CAD build for the part. Positions are in the model's coordinates, mm. A direction names the side the tool comes from. Coordinates: 2 decimals unless noted, no trailing zeros. Order: outer loops, then holes, each group sorted by start corner. A loop starts at its lowest first (then second) coordinate and runs counter-clockwise, first axis right, second up.
Autodesk Inventor part; units mm, degrees
ref_plane "YZ Plane" through (0, 0, 0) normal (1, 0, 0) x (0, 1, 0)
ref_plane "XZ Plane" through (0, 0, 0) normal (0, 1, 0) x (-1, 0, 0)
ref_plane "XY Plane" through (0, 0, 0) normal (0, 0, 1) x (1, 0, 0)
sketch "Sketch1" plane through (0, 0, 0) normal (0, 1, 0) x (-1, 0, 0)
  circle A0 centre (0, 0) radius 60
  dimension "d0" = 120
extrude "Extrusion1" add sketch "Sketch1" along normal blind 8
sketch "Sketch2" plane through (0, 8, 0) normal (0, 1, 0) x (1, 0, 0)
  circle A0 centre (-54, 0) radius 4
  circle A1 centre (-54, 0) radius 2.5
  circle A2 centre (0, -54) radius 4
  circle A3 centre (0, -54) radius 2.5
  circle A4 centre (54, 0) radius 4
  circle A5 centre (54, 0) radius 2.5
  circle A6 centre (0, 54) radius 4
  circle A7 centre (0, 54) radius 2.5
  point P0 (0, 0)
  dimension "d3" = 8
  dimension "d4" = 5
  dimension "d5" = 8
  dimension "d6" = 5
  dimension "d7" = 8
  dimension "d8" = 5
  dimension "d9" = 8
  dimension "d10" = 5
extrude "Extrusion2" cut sketch "Sketch2" against normal blind 8 contours A1 | A3 | A5 | A7
sketch "Sketch3" plane through (0, 8, 0) normal (0, 1, 0) x (1, 0, 0)
  circle A0 centre (-54, 0) radius 2.5
  circle A1 centre (-54, 0) radius 4
  circle A2 centre (-54, 0) radius 2.5
  circle A3 centre (0, 54) radius 2.5
  circle A4 centre (0, 54) radius 4
  circle A5 centre (0, 54) radius 2.5
  circle A6 centre (54, 0) radius 2.5
  circle A7 centre (54, 0) radius 4
  circle A8 centre (54, 0) radius 2.5
  circle A9 centre (0, -54) radius 4
  circle A10 centre (0, -54) radius 2.5
  point P0 (0, 0)
  dimension "d13" = 8
  dimension "d14" = 8
  dimension "d15" = 5
  dimension "d16" = 8
  dimension "d17" = 5
  dimension "d18" = 8
extrude "Extrusion3" cut sketch "Sketch3" against normal blind 3
sketch "Sketch4" plane through (0, 8, 0) normal (0, 1, 0) x (1, 0, 0)
  circle A0 centre (0, 0) radius 47.5
  circle A1 centre (0, 0) radius 45
  line L0 (0, 0) -> (-10, 0)
  line L1 (-10, 0) -> (-10, -9)
  line L2 (-10, -9) -> (0, -9)
  line L3 (0, -9) -> (0, 0)
  line L4 (0, -9) -> (10, -9)
  line L5 (10, -9) -> (10, 0)
  line L6 (10, 0) -> (0, 0)
  line L7 (0, 0) -> (0, -9)
  line L8 (-10, -9) -> (10, -9)
  line L9 (10, -9) -> (10, -16)
  line L10 (10, -16) -> (-10, -16)
  line L11 (-10, -16) -> (-10, -9)
  dimension "d21" = 95
  dimension "d22" = 90
  dimension "d23" = 10
  dimension "d24" = 9
  dimension "d25" = 10
  dimension "d26" = 7
extrude "Extrusion4" add sketch "Sketch4" along normal blind 10 contours A0
sketch "Sketch5" plane through (0, 8, 0) normal (0, 1, 0) x (1, 0, 0)
  line L0 (0, 0) -> (-10, 0)
  line L1 (-10, 0) -> (-10, -9)
  line L2 (-10, -9) -> (0, -9)
  line L3 (0, -9) -> (0, 0)
  line L4 (-10, -9) -> (10, -9)
  line L5 (10, -9) -> (10, -16)
  line L6 (10, -16) -> (-10, -16)
  line L7 (-10, -16) -> (-10, -9)
  line L8 (-10, -9) -> (10, -9)
  line L9 (10, -9) -> (10, 31)
  line L10 (10, 31) -> (-10, 31)
  line L11 (-10, 31) -> (-10, -9)
  line L12 (-10, 31) -> (-2, 31)
  line L13 (-2, 31) -> (-2, 38.36)
  line L14 (-2, 38.36) -> (-10, 38.36)
  line L15 (-10, 38.36) -> (-10, 31)
  line L16 (-10, 31) -> (10, 31)
  line L17 (10, 31) -> (10, 39)
  line L18 (10, 39) -> (-10, 39)
  line L19 (-10, 39) -> (-10, 31)
  line L20 (-10, -9) -> (10, -9)
  line L21 (10, -9) -> (10, -17)
  line L22 (10, -17) -> (-10, -17)
  line L23 (-10, -17) -> (-10, -9)
  dimension "d29" = 10
  dimension "d30" = 9
  dimension "d31" = 20
  dimension "d32" = 7
  dimension "d33" = 40
  dimension "d34" = 8
  dimension "d35" = 8
  dimension "d36" = 8
extrude "Extrusion5" add sketch "Sketch5" along normal blind 28 contours L4 L5 L6 L7 L2 | L15 L14 L13 L10 | L6 L21 L22 L23 | L13 L14 L19 L18 L17 L10
sketch "Sketch6" plane through (0, 36, 0) normal (0, 1, 0) x (1, 0, 0)
  line L0 (10, -17) -> (-10, -17)
  line L1 (-10, -9) -> (10, -9)
  line L2 (0, -17) -> (-4, -17)
  line L3 (-4, -17) -> (-4, -9)
  line L4 (-4, -9) -> (0, -9)
  line L5 (0, -9) -> (0, -17)
  line L6 (0, -17) -> (4, -17)
  line L7 (4, -17) -> (4, -9)
  line L8 (4, -9) -> (0, -9)
  line L9 (0, -9) -> (0, -17)
  point P0 (0, 0)
  dimension "d39" = 4
  dimension "d40" = 4
extrude "Extrusion6" cut sketch "Sketch6" against normal blind 28
sketch "Sketch7" plane through (0, 36, 0) normal (0, 1, 0) x (1, 0, 0)
  line L0 (-10, -17) -> (-4, -17)
  line L1 (4, -9) -> (10, -9)
  line L2 (-4, -17) -> (4, -17)
  line L3 (4, -17) -> (4, -9)
  line L4 (4, -9) -> (-4, -9)
  line L5 (-4, -9) -> (-4, -17)
  point P0 (0, 0)
extrude "Extrusion7" add sketch "Sketch7" against normal blind 22
sketch "Sketch8" plane through (0, 36, 0) normal (0, 1, 0) x (1, 0, 0)
  line L0 (-4, -17) -> (-10, -17)
  line L1 (10, -17) -> (10, -9)
  line L2 (-10, -17) -> (10, -17)
  line L3 (10, -17) -> (10, -15)
  line L4 (10, -15) -> (-10, -15)
  line L5 (-10, -15) -> (-10, -17)
  line L6 (-4, -9) -> (4, -9)
  line L7 (0, -9) -> (-5, -9)
  line L8 (-5, -9) -> (-5, -17)
  line L9 (-5, -17) -> (0, -17)
  line L10 (0, -17) -> (0, -9)
  line L11 (-10, -17) -> (10, -17)
  line L12 (0, -9) -> (5, -9)
  line L13 (5, -9) -> (5, -17)
  line L14 (5, -17) -> (0, -17)
  line L15 (0, -17) -> (0, -9)
  circle A0 centre (-5, -15) radius 2
  circle A1 centre (5, -15) radius 2
  line L16 (-10, 31) -> (-10, 39)
  line L17 (10, 39) -> (10, 31)
  line L18 (-10, 39) -> (10, 39)
  line L19 (10, 39) -> (10, 37)
  line L20 (10, 37) -> (-10, 37)
  line L21 (-10, 37) -> (-10, 39)
  line L22 (10, 31) -> (-10, 31)
  line L23 (-10, 39) -> (10, 39)
  line L24 (0, 31) -> (-5, 31)
  line L25 (-5, 31) -> (-5, 39)
  line L26 (-5, 39) -> (0, 39)
  line L27 (0, 39) -> (0, 31)
  line L28 (0, 31) -> (5, 31)
  line L29 (5, 31) -> (5, 39)
  line L30 (5, 39) -> (0, 39)
  line L31 (0, 39) -> (0, 31)
  circle A2 centre (-5, 37) radius 2
  circle A3 centre (5, 37) radius 2
  point P0 (0, 0)
  dimension "d45" = 2
  dimension "d46" = 5
  dimension "d47" = 5
  dimension "d48" = 4
  dimension "d49" = 4
  dimension "d50" = 2
  dimension "d51" = 4
  dimension "d52" = 4
extrude "Extrusion8" cut sketch "Sketch8" against normal blind 10 contours A0 L4 L8 | L8 L4 A0 | L8 A0 L4 | L4 A0 L8 | A1 L4 L13 | L13 L4 A1 | L13 A1 L4 | L4 A1 L13 | A2 L25 L20 | L20 L25 A2 | L25 L20 A2 | A2 L20 L25 | A3 L20 L29 | L29 L20 A3 | A3 L29 L20 | A3 L20 L29
sketch "Sketch9" plane through (0, 36, 0) normal (0, 1, 0) x (1, 0, 0)
  line L0 (-10, -17) -> (-5, -17)
  line L1 (10, -9) -> (-10, -9)
  line L2 (-10, -17) -> (10, -17)
  line L3 (10, -17) -> (10, -9)
  line L4 (10, -9) -> (-10, -9)
  line L5 (-10, -9) -> (-10, -17)
  line L6 (10, 31) -> (10, 39)
  line L7 (-10, 31) -> (10, 31)
  line L8 (10, 31) -> (10, 39)
  line L9 (10, 39) -> (-10, 39)
  line L10 (-10, 39) -> (-10, 31)
  point P0 (0, 0)
extrude "Extrusion9" cut sketch "Sketch9" against normal blind 28
sketch "Sketch10" plane through (0, 8, 0) normal (0, 1, 0) x (1, 0, 0)
  line L0 (0, 0) -> (-10, 0)
  line L1 (-10, 0) -> (-10, 36.5)
  line L2 (-10, 36.5) -> (0, 36.5)
  line L3 (0, 36.5) -> (0, 0)
  line L4 (-10, 0) -> (0, 0)
  line L5 (0, 0) -> (0, -16.9)
  line L6 (0, -16.9) -> (-10, -16.9)
  line L7 (-10, -16.9) -> (-10, 0)
  line L8 (0, -16.9) -> (10, -16.9)
  line L9 (10, -16.9) -> (10, 36.5)
  line L10 (10, 36.5) -> (0, 36.5)
  line L11 (0, 36.5) -> (0, -16.9)
  line L12 (-10, -16.9) -> (10, -16.9)
  line L13 (10, -16.9) -> (10, -10.9)
  line L14 (10, -10.9) -> (-10, -10.9)
  line L15 (-10, -10.9) -> (-10, -16.9)
  line L16 (-10, 36.5) -> (10, 36.5)
  line L17 (10, 36.5) -> (10, 30.5)
  line L18 (10, 30.5) -> (-10, 30.5)
  line L19 (-10, 30.5) -> (-10, 36.5)
  line L20 (-10, -16.9) -> (-4, -16.9)
  line L21 (-4, -16.9) -> (-4, -10.9)
  line L22 (-4, -10.9) -> (-10, -10.9)
  line L23 (-10, -10.9) -> (-10, -16.9)
  line L24 (10, -16.9) -> (4, -16.9)
  line L25 (4, -16.9) -> (4, -10.9)
  line L26 (4, -10.9) -> (10, -10.9)
  line L27 (10, -10.9) -> (10, -16.9)
  dimension "d57" = 10
  dimension "d58" = 36.5
  dimension "d59" = 16.9
  dimension "d60" = 10
  dimension "d61" = 6
  dimension "d62" = 6
  dimension "d63" = 6
  dimension "d64" = 6
extrude "Extrusion10" add sketch "Sketch10" along normal blind 10 contours L18 L1 L2 L3 | L3 L10 L9 L18 | L14 L21 L6 L7 | L14 L9 L8 L25
sketch "Sketch11" plane through (0, 18, 0) normal (0, 1, 0) x (1, 0, 0)
  line L0 (-10, 30.5) -> (10, 30.5)
  line L1 (10, 36.5) -> (-10, 36.5)
  line L2 (-10, 30.5) -> (10, 30.5)
  line L3 (10, 30.5) -> (10, 36.5)
  line L4 (10, 36.5) -> (-10, 36.5)
  line L5 (-10, 36.5) -> (-10, 30.5)
  line L6 (-10, -16.9) -> (-4, -16.9)
  line L7 (10, -10.9) -> (4, -10.9)
  line L8 (-10, -16.9) -> (10, -16.9)
  line L9 (10, -16.9) -> (10, -10.9)
  line L10 (10, -10.9) -> (-10, -10.9)
  line L11 (-10, -10.9) -> (-10, -16.9)
  point P0 (0, 0)
extrude "Extrusion11" add sketch "Sketch11" along normal blind 16.7
sketch "Sketch12" plane through (0, 34.7, 0) normal (0, 1, 0) x (1, 0, 0)
  line L0 (10, -16.9) -> (10, -10.9)
  line L1 (-10, -16.9) -> (10, -16.9)
  line L2 (10, -16.9) -> (10, -14.35)
  line L3 (10, -14.35) -> (-10, -14.35)
  line L4 (-10, -14.35) -> (-10, -16.9)
  line L5 (10, 30.5) -> (10, 36.5)
  line L6 (-10, 36.5) -> (10, 36.5)
  line L7 (10, 36.5) -> (10, 33.95)
  line L8 (10, 33.95) -> (-10, 33.95)
  line L9 (-10, 33.95) -> (-10, 36.5)
  line L10 (0, -16.9) -> (5.05, -16.9)
  line L11 (5.05, -16.9) -> (5.05, -14.35)
  line L12 (5.05, -14.35) -> (0, -14.35)
  line L13 (0, -14.35) -> (0, -16.9)
  line L14 (0, -16.9) -> (-5.05, -16.9)
  line L15 (-5.05, -16.9) -> (-5.05, -14.35)
  line L16 (-5.05, -14.35) -> (0, -14.35)
  line L17 (0, -14.35) -> (0, -16.9)
  line L18 (10, 36.5) -> (-10, 36.5)
  line L19 (0, 36.5) -> (-5.05, 36.5)
  line L20 (-5.05, 36.5) -> (-5.05, 33.95)
  line L21 (-5.05, 33.95) -> (0, 33.95)
  line L22 (0, 33.95) -> (0, 36.5)
  line L23 (0, 36.5) -> (5.05, 36.5)
  line L24 (5.05, 36.5) -> (5.05, 33.95)
  line L25 (5.05, 33.95) -> (0, 33.95)
  line L26 (0, 33.95) -> (0, 36.5)
  circle A0 centre (-5.05, -14.35) radius 1.35
  circle A1 centre (5.05, -14.35) radius 1.35
  circle A2 centre (-5.05, 33.95) radius 1.35
  circle A3 centre (5.05, 33.95) radius 1.35
  point P0 (0, 0)
  dimension "d69" = 2.55
  dimension "d70" = 2.55
  dimension "d71" = 5.05
  dimension "d72" = 5.05
  dimension "d73" = 5.05
  dimension "d74" = 5.05
  dimension "d75" = 2.7
  dimension "d76" = 2.7
  dimension "d77" = 2.7
  dimension "d78" = 2.7
extrude "Extrusion12" cut sketch "Sketch12" against normal blind 10 contours A1 L11 L3 | L3 A1 | A1 L3 L11 | A0 L3 L15 | L15 L3 A0 | L3 A0 | A3 L8 | L8 L24 A3 | L8 A3 L24 | A2 L8 | L8 L20 A2 | L20 L8 A2
thread "Thread1"
thread "Thread2"
thread "Thread3"
thread "Thread4"
sketch "Sketch13" plane through (0, 18, 0) normal (0, 1, 0) x (1, 0, 0)
  circle A0 centre (0, 0) radius 45
  circle A1 centre (0, 0) radius 47.5
extrude "Extrusion13" cut sketch "Sketch13" against normal blind 47.3
sketch "Sketch14" plane through (0, 8, 0) normal (0, 1, 0) x (1, 0, 0)
  circle A0 centre (0, 0) radius 45
  circle A1 centre (0, 0) radius 47.5
extrude "Extrusion14" add sketch "Sketch14" along normal blind 42.5
sketch "Sketch16" plane through (0, 50.5, 0) normal (0, 1, 0) x (1, 0, 0)
  circle A0 centre (0, 0) radius 45
  circle A1 centre (0, 0) radius 47.5
extrude "Extrusion15" cut sketch "Sketch16" against normal blind 42.5
sketch "Sketch17" plane through (0, 0, 0) normal (0, -1, 0) x (1, 0, 0)
  circle A0 centre (0, 0) radius 47.5
  circle A1 centre (0, 0) radius 45
extrude "Extrusion16" add sketch "Sketch17" against normal blind 8
sketch "Sketch18" plane through (0, 8, 0) normal (0, 1, 0) x (1, 0, 0)
  circle A0 centre (0, 0) radius 47.5
  circle A1 centre (0, 0) radius 45
  dimension "d97" = 95
  dimension "d98" = 90
extrude "Extrusion17" add sketch "Sketch18" along normal blind 42.5
properties part number "NBase Part"
1) Which spindle directions (+Z, -Z, +X, -X, +Y, -Y) get a long thin tool onto all of the face, cutting with end or side? Do faces 3 (the flat face through (-52, 5, -2)), 4 (the flat face through (-4, 13, 14)). Say none if no direction does.
2) Slice it at A-A (y = 28.5). List the corners of the cut face in (x, z), plus the area to 3 significant figures.
3) Two-plate mould, pull along Z, no slides. Class faces 1 (the flat face through (0, 21, -30.5)), 2 (the cylindrical face through (-10.3, 28.95, -46.37)): released by +Z, released by -Z, zero draft, split by the parting line, or undercut.
4) Slice it at D-D (z = -54). List the corners of the cut face in (x, y), plus the area to 3 significant figures.
5) Drill centre lines: probe 1 along Z at (x, y) = (0, 6.3); probe 2 along Z at (x, y) = (-9.5, 21.5); probe 3 along Z at (x, y) = (5, 32). Where is each one in solid material? Low to high.
6) Pin check, flat tips, straight feed: P1, Ø12, axis at x = -40.5, y = 25, coming from the -Z side; P2, Ø1.5, axis at y = 41, z = 2, coming from the -X side; P3, Ø10, axis at x = 15, z = 18, coming from the +Y side. Stop position of each tip, or through.
7) Slice it at C-C (z = 0). List the corners of the cut face in (x, y).
8) Slice it at B-B (y = 14). List the corners of the cut face in (x, z).
Worked out:
1. face 3: +Y
1. face 4: none
2. outline: circle Ø95 at (0, 0); (-10, -36.5) - (10, -36.5) - (10, -30.5) - (-10, -30.5) - close; (-10, 10.9) - (10, 10.9) - (10, 16.9) - (-10, 16.9) - close; hole circle Ø90 at (0, 0); hole circle Ø2.7 at (-5.05, -33.95); hole circle Ø2.7 at (-5.05, 14.35); hole circle Ø2.7 at (5.05, -33.95); hole circle Ø2.7 at (5.05, 14.35)
2. area: 944 mm2
3. face 1: undercut
3. face 2: split by the parting line
4. outline: (-26.15, 0) - (-2.5, 0) - (-2.5, 5) - (-4, 5) - (-4, 8) - (-26.15, 8) - close; (2.5, 0) - (26.15, 0) - (26.15, 8) - (4, 8) - (4, 5) - (2.5, 5) - close
4. area: 369 mm2
5. probe 1: z = -60 to -58, -50 to 50, 58 to 60
5. probe 2: z = -46.54 to -43.99, -36.5 to -30.5, 10.9 to 16.9, 43.99 to 46.54
5. probe 3: z = -47.24 to -44.72, -36.5 to -35.3, -32.6 to -30.5, 10.9 to 13, 15.7 to 16.9, 44.72 to 47.24
6. P1: stops at z = -32.65
6. P2: stops at x = -47.48
6. P3: stops at y = 8
7. outline: (-60, 0) - (-56.5, 0) - (-56.5, 5) - (-58, 5) - (-58, 8) - (-60, 8) - close; (-51.5, 0) - (51.5, 0) - (51.5, 5) - (50, 5) - (50, 8) - (47.5, 8) - (47.5, 50.5) - (45, 50.5) - (45, 8) - (-45, 8) - (-45, 50.5) - (-47.5, 50.5) - (-47.5, 8) - (-50, 8) - (-50, 5) - (-51.5, 5) - close; (56.5, 0) - (60, 0) - (60, 8) - (58, 8) - (58, 5) - (56.5, 5) - close
8. outline: circle Ø95 at (0, 0); (-10, -36.5) - (10, -36.5) - (10, -30.5) - (-10, -30.5) - close; (-10, 10.9) - (-4, 10.9) - (-4, 16.9) - (-10, 16.9) - close; (4, 10.9) - (10, 10.9) - (10, 16.9) - (4, 16.9) - close; hole circle Ø90 at (0, 0)
